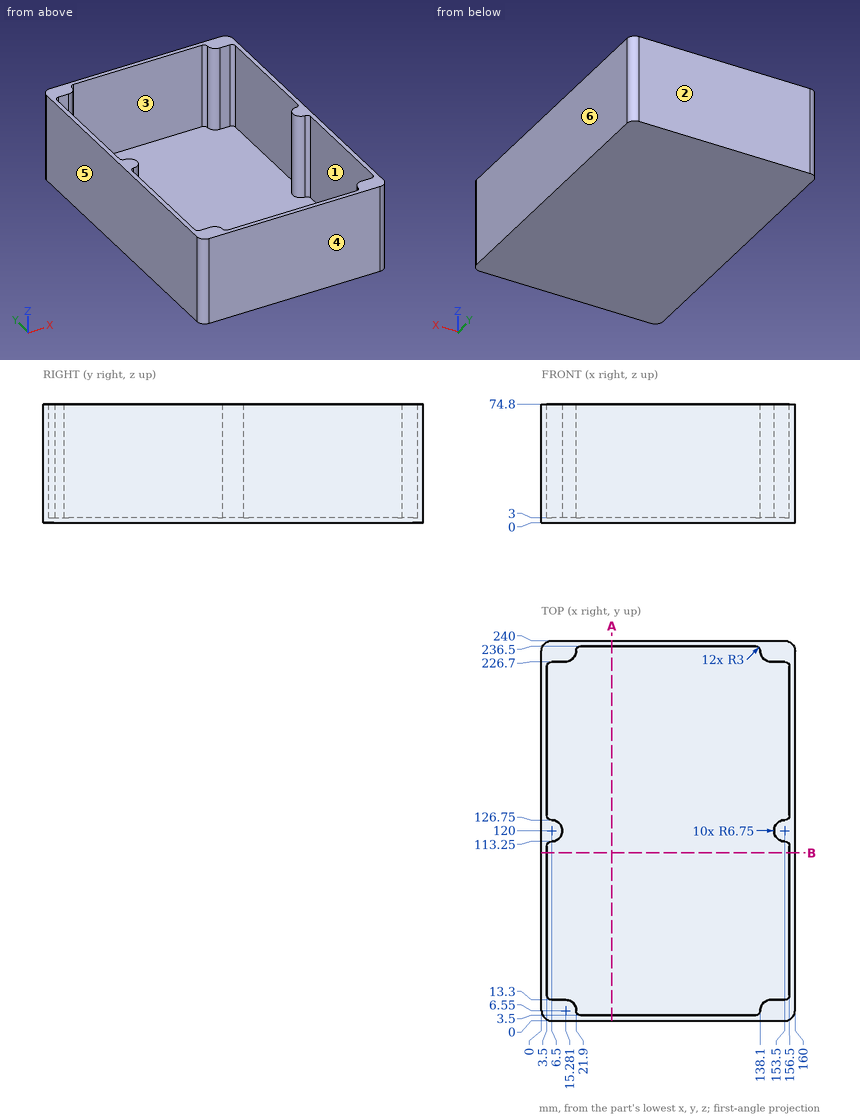
Can you work these out from the drawing? Everything is in mm from the part's minimum corner. A direction names the side the tool comes from. Round coordinates to 2 decimals unless told otherwise and drop trailing zeros. Loops run counter-clockwise (first coordinate to the right, second up) from the corner with the lowest first, then second, coordinate; pieces in that order, holes last. Notation, with made-up numbers: (-1.75, 4.25) -> (19.25, 4.25) arc R14 cw to (19.25, 13.25) -> close; hole circle Ø10 at (30, 77). An arc over 180 degrees is marked (long way). Answer in a Markdown table with one row per item.
Item 1: We'd pull the mould along X, two halves only. Please class the marked faces 3, 4, 5 and 6: released by +X, released by -X, zero draft, split by the parting line, or undercut.
Answer block:
| item | result |
|---|---|
| face 3 | undercut |
| face 4 | zero draft |
| face 5 | released by -X |
| face 6 | released by +X |
Item 2: Suppose I cut it at A-A, the plane x = 44.5. List the corners of the cut face in (y, z) for me.
Answer block:
| item | result |
|---|---|
| outline | (0, 0) -> (240, 0) -> (240, 74.8) -> (236.5, 74.8) -> (236.5, 3) -> (3.5, 3) -> (3.5, 74.8) -> (0, 74.8) -> close |
Item 3: Suppose I cut it at B-B, the plane y = 106. List the corners of the cut face in (x, z) for me.
Answer block:
| item | result |
|---|---|
| outline | (0, 0) -> (160, 0) -> (160, 74.8) -> (156.5, 74.8) -> (156.5, 3) -> (3.5, 3) -> (3.5, 74.8) -> (0, 74.8) -> close |
Item 4: If I drill on probe 1 along Y at (x, z) = (35, 48); probe 2 along X at (y, z) = (80, 69); probe 3 along Z at (x, y) = (52, 126.5), over which ranges is the centre line in solid material (lowest first)?
Answer block:
| item | result |
|---|---|
| probe 1 | 0 to 3.5, 236.5 to 240 |
| probe 2 | 0 to 3.5, 156.5 to 160 |
| probe 3 | 0 to 3 |
Item 5: On a 3-axis mill with a long thin cutter (end or side, diameter ignored), from which of +Z, -Z, +X, -X, +Y, -Y can I reach the whole of each face in a straight line? I mean the marked faces 1 and 2. Say none if no direction works.
Answer block:
| item | result |
|---|---|
| face 1 | +Z |
| face 2 | +Z, -Z, +X, -X, +Y |
Item 6: Will this pin go through, and if not, where does the flat tip stop? P1, Ø1, axis at x = 107, y = 210.5, coming from the +Z side.
Answer block:
| item | result |
|---|---|
| P1 | z = 3 |
